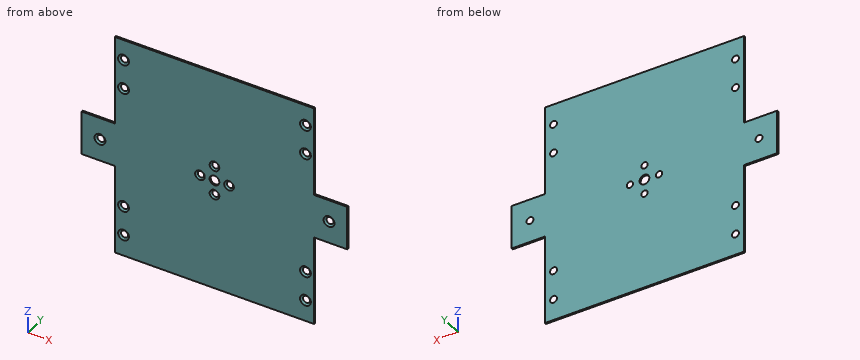
from build123d import *

# Parameters (mm, degrees)
BOSS_EXTRUDE1_DEPTH                            = 1.0668
CSK_FOR_6_FLAT_HEAD_MACHINE_SCREW_2_COUNT      = 2
CSK_FOR_6_FLAT_HEAD_MACHINE_SCREW_2_PITCH      = 117.475
CSK_FOR_6_FLAT_HEAD_MACHINE_SCREW_3_COUNT      = 2
CSK_FOR_6_FLAT_HEAD_MACHINE_SCREW_3_PITCH      = 167.102910264
CSK_FOR_6_FLAT_HEAD_MACHINE_SCREW_4_COUNT      = 2
CSK_FOR_6_FLAT_HEAD_MACHINE_SCREW_4_PITCH      = 118.84025
CSK_FOR_6_FLAT_HEAD_MACHINE_SCREW_5_COUNT      = 2
CSK_FOR_6_FLAT_HEAD_MACHINE_SCREW_5_PITCH      = 120.377583757
CSK_FOR_6_FLAT_HEAD_MACHINE_SCREW_6_COUNT      = 2
CSK_FOR_6_FLAT_HEAD_MACHINE_SCREW_6_PITCH      = 98.298
CSK_FOR_6_FLAT_HEAD_MACHINE_SCREW_7_COUNT      = 2
CSK_FOR_6_FLAT_HEAD_MACHINE_SCREW_7_PITCH      = 154.225495543
CSK_FOR_6_FLAT_HEAD_MACHINE_SCREW_8_COUNT      = 2
CSK_FOR_6_FLAT_HEAD_MACHINE_SCREW_8_PITCH      = 19.177
CSK_FOR_6_FLAT_HEAD_MACHINE_SCREW_9_COUNT      = 2
CSK_FOR_6_FLAT_HEAD_MACHINE_SCREW_9_PITCH      = 60.937464766
CSK_FOR_6_FLAT_HEAD_MACHINE_SCREW_10_COUNT     = 2
CSK_FOR_6_FLAT_HEAD_MACHINE_SCREW_10_PITCH     = 146.616377774
SKETCH4_R                                      = 3.175
CUT_EXTRUDE1_DEPTH                             = 113.951767191
CSK_FOR_M3_FLAT_HEAD_MACHINE_SCREW2_AT_2_COUNT = 2
CSK_FOR_M3_FLAT_HEAD_MACHINE_SCREW2_AT_2_PITCH = 19
CSK_FOR_M3_FLAT_HEAD_MACHINE_SCREW2_AT_3_COUNT = 2
CSK_FOR_M3_FLAT_HEAD_MACHINE_SCREW2_AT_3_PITCH = 13.435028843
CSK_FOR_M3_FLAT_HEAD_MACHINE_SCREW2_AT_4_COUNT = 2
CSK_FOR_M3_FLAT_HEAD_MACHINE_SCREW2_AT_4_PITCH = 13.435028843


with BuildPart() as part:
    # Sketch1 → Boss-Extrude1 (new body)
    with BuildSketch(Plane(origin=(0, 0, 0), x_dir=(1, 0, 0), z_dir=(0, 1, 0))):
        Polygon((-65.0875, 72.35825), (65.0875, 72.35825), (65.0875, 14.25575), (86.725125, 14.25575), (86.725125, -14.25575), (65.0875, -14.25575), (65.0875, -72.35825), (-65.0875, -72.35825), (-65.0875, -14.25575), (-86.725125, -14.25575), (-86.725125, 14.25575), (-65.0875, 14.25575), align=None)
    extrude(amount=BOSS_EXTRUDE1_DEPTH)

    # Sketch2 → CSK for #6 Flat Head Machine Screw (100)1 (revolve, cut)
    with BuildSketch(Plane(origin=(-59.420125, 0, 58.9597584), x_dir=(0, 0, -1), z_dir=(1, 0, 0))):
        Polygon((0, 0), (0, 1.0668), (1.89865, 1.0668), (1.89865, 1.380025208), (3.5433, 0), align=None)
    csk_for_6_flat_head_machine_screw_100 = revolve(axis=Axis((-59.420125, -6.35, 58.9597584), (0, 1, 0)), mode=Mode.SUBTRACT)

    # CSK for _6 Flat Head Machine Screw _ 2: CSK for #6 Flat Head Machine Screw (100)1 ×2
    with Locations(*[(0, 0, -i * CSK_FOR_6_FLAT_HEAD_MACHINE_SCREW_2_PITCH) for i in range(1, CSK_FOR_6_FLAT_HEAD_MACHINE_SCREW_2_COUNT)]):
        add(csk_for_6_flat_head_machine_screw_100, mode=Mode.SUBTRACT)

    # CSK for _6 Flat Head Machine Screw _ 3: CSK for #6 Flat Head Machine Screw (100)1 ×2
    with Locations(*[Vector(0.7111800136357133, 0, -0.7030099488663775) * (i * CSK_FOR_6_FLAT_HEAD_MACHINE_SCREW_3_PITCH) for i in range(1, CSK_FOR_6_FLAT_HEAD_MACHINE_SCREW_3_COUNT)]):
        add(csk_for_6_flat_head_machine_screw_100, mode=Mode.SUBTRACT)

    # CSK for _6 Flat Head Machine Screw _ 4: CSK for #6 Flat Head Machine Screw (100)1 ×2
    with Locations(*[(i * CSK_FOR_6_FLAT_HEAD_MACHINE_SCREW_4_PITCH, 0, 0) for i in range(1, CSK_FOR_6_FLAT_HEAD_MACHINE_SCREW_4_COUNT)]):
        add(csk_for_6_flat_head_machine_screw_100, mode=Mode.SUBTRACT)

    # CSK for _6 Flat Head Machine Screw _ 5: CSK for #6 Flat Head Machine Screw (100)1 ×2
    with Locations(*[Vector(0.9872290694888833, 0, -0.15930713843426378) * (i * CSK_FOR_6_FLAT_HEAD_MACHINE_SCREW_5_PITCH) for i in range(1, CSK_FOR_6_FLAT_HEAD_MACHINE_SCREW_5_COUNT)]):
        add(csk_for_6_flat_head_machine_screw_100, mode=Mode.SUBTRACT)

    # CSK for _6 Flat Head Machine Screw _ 6: CSK for #6 Flat Head Machine Screw (100)1 ×2
    with Locations(*[(0, 0, -i * CSK_FOR_6_FLAT_HEAD_MACHINE_SCREW_6_PITCH) for i in range(1, CSK_FOR_6_FLAT_HEAD_MACHINE_SCREW_6_COUNT)]):
        add(csk_for_6_flat_head_machine_screw_100, mode=Mode.SUBTRACT)

    # CSK for _6 Flat Head Machine Screw _ 7: CSK for #6 Flat Head Machine Screw (100)1 ×2
    with Locations(*[Vector(0.7705616349723654, 0, -0.6373654891102241) * (i * CSK_FOR_6_FLAT_HEAD_MACHINE_SCREW_7_PITCH) for i in range(1, CSK_FOR_6_FLAT_HEAD_MACHINE_SCREW_7_COUNT)]):
        add(csk_for_6_flat_head_machine_screw_100, mode=Mode.SUBTRACT)

    # CSK for _6 Flat Head Machine Screw _ 8: CSK for #6 Flat Head Machine Screw (100)1 ×2
    with Locations(*[(0, 0, -i * CSK_FOR_6_FLAT_HEAD_MACHINE_SCREW_8_PITCH) for i in range(1, CSK_FOR_6_FLAT_HEAD_MACHINE_SCREW_8_COUNT)]):
        add(csk_for_6_flat_head_machine_screw_100, mode=Mode.SUBTRACT)

    # CSK for _6 Flat Head Machine Screw _ 9: CSK for #6 Flat Head Machine Screw (100)1 ×2
    with Locations(*[Vector(-0.2526975820055066, 0, -0.9675453126590869) * (i * CSK_FOR_6_FLAT_HEAD_MACHINE_SCREW_9_PITCH) for i in range(1, CSK_FOR_6_FLAT_HEAD_MACHINE_SCREW_9_COUNT)]):
        add(csk_for_6_flat_head_machine_screw_100, mode=Mode.SUBTRACT)

    # CSK for _6 Flat Head Machine Screw _ 10: CSK for #6 Flat Head Machine Screw (100)1 ×2
    with Locations(*[Vector(0.915579842020543, 0, -0.40213623672287674) * (i * CSK_FOR_6_FLAT_HEAD_MACHINE_SCREW_10_PITCH) for i in range(1, CSK_FOR_6_FLAT_HEAD_MACHINE_SCREW_10_COUNT)]):
        add(csk_for_6_flat_head_machine_screw_100, mode=Mode.SUBTRACT)

    # Sketch4 → Cut-Extrude1 (cut, through all)
    with BuildSketch(Plane.XZ):
        with Locations(Location((0, 0, 0), (0, 0, 270))):
            Circle(SKETCH4_R)
    extrude(amount=-CUT_EXTRUDE1_DEPTH, mode=Mode.SUBTRACT)

    # Sketch5 → CSK for M3 Flat Head Machine Screw2 (revolve, cut)
    with BuildSketch(Plane(origin=(9.5, 0, 0), x_dir=(0, 0, -1), z_dir=(1, 0, 0))):
        Polygon((0, 0), (0, 1.0668), (1.7, 1.0668), (1.7, 1.45), (3.15, 0), align=None)
    csk_for_m3_flat_head_machine_screw2 = revolve(axis=Axis((9.5, -6.35, 0), (0, 1, 0)), mode=Mode.SUBTRACT)

    # CSK for M3 Flat Head Machine Screw2 at 2: CSK for M3 Flat Head Machine Screw2 ×2
    with Locations(*[(-i * CSK_FOR_M3_FLAT_HEAD_MACHINE_SCREW2_AT_2_PITCH, 0, 0) for i in range(1, CSK_FOR_M3_FLAT_HEAD_MACHINE_SCREW2_AT_2_COUNT)]):
        add(csk_for_m3_flat_head_machine_screw2, mode=Mode.SUBTRACT)

    # CSK for M3 Flat Head Machine Screw2 at 3: CSK for M3 Flat Head Machine Screw2 ×2
    with Locations(*[Vector(-0.7071067811865486, 0, -0.7071067811865466) * (i * CSK_FOR_M3_FLAT_HEAD_MACHINE_SCREW2_AT_3_PITCH) for i in range(1, CSK_FOR_M3_FLAT_HEAD_MACHINE_SCREW2_AT_3_COUNT)]):
        add(csk_for_m3_flat_head_machine_screw2, mode=Mode.SUBTRACT)

    # CSK for M3 Flat Head Machine Screw2 at 4: CSK for M3 Flat Head Machine Screw2 ×2
    with Locations(*[Vector(-0.7071067811865486, 0, 0.7071067811865466) * (i * CSK_FOR_M3_FLAT_HEAD_MACHINE_SCREW2_AT_4_PITCH) for i in range(1, CSK_FOR_M3_FLAT_HEAD_MACHINE_SCREW2_AT_4_COUNT)]):
        add(csk_for_m3_flat_head_machine_screw2, mode=Mode.SUBTRACT)


solid = part.part
Could you check a few things on this model? Use its own coordinates, in mm. Give positions to 0.01 mm unless a question says otherwise; leave off trailing zeros. Order: outer loops, then holes, each group sorted by start corner. A loop starts at its lowest first (then second) coordinate and runs counter-clockwise, first axis right, second up. Notation, with made-up numbers: (42.5, 62.5) - (55.5, 62.5) arc R19 ccw to (55.5, 66.5) - close; hole circle Ø2 at (-7, -7.75). An arc over 180 degrees is marked (long way). One line per item, written item: value. Start each with the question number.
1. If I drill on probe 1 along X at (y, z) = (0.8, 0) (3 decimals); probe 2 along X at (y, z) = (0.3, 0) (3 decimals); probe 3 along Z at (x, y) = (-67, 0.2), over which ranges is the centre line in solid material (lowest first)?
2. For P1, Ø0.5, axis at y = 0.5, z = -36.5, coming from the +X side, with a flat end and sliding along its axis, tell me the tip position at first contact or that it passes through.
3. Imagine slicing it at C-C on y = 0.35. Give the number of separate pieces and of enclosed holes in the cut face, plus the area to 3 significant figures.
4. Imagine slicing it at D-D on z = 46. List the corners of the cut face in (x, y) for me.
5. Imagine slicing it at A-A on z = 9.5. List the corners of the cut face in (x, y) for me, plus the area to 3 significant figures.
6. Imagine slicing it at B-B on x = -9.5. List the corners of the cut face in (y, z) for me, plus the area to 3 significant figures.
Values:
1. probe 1: -86.725 to -77.409, -72.229 to -11.85, -7.15 to -3.175, 3.175 to 7.15, 11.85 to 72.229, 77.409 to 86.725
1. probe 2: -86.725 to -78.005, -71.633 to -12.35, -6.65 to -3.175, 3.175 to 6.65, 12.35 to 71.633, 78.005 to 86.725
1. probe 3: -14.26 to 14.26
2. P1: x = 65.09
3. separate pieces: 1
3. enclosed holes: 15
3. area: 19,600 mm²
4. outline: (-65.09, 0) - (65.09, 0) - (65.09, 1.07) - (-65.09, 1.07) - close
5. outline: (-86.73, 0) - (-3.15, 0) - (-2.08, 1.07) - (-86.73, 1.07) - close; (2.08, 1.07) - (3.15, 0) - (86.73, 0) - (86.73, 1.07) - close
5. area: 179 mm²
6. outline: (0, -72.36) - (1.07, -72.36) - (1.07, -2.08) - (0, -3.15) - close; (0, 3.15) - (1.07, 2.08) - (1.07, 72.36) - (0, 72.36) - close
6. area: 149 mm²
